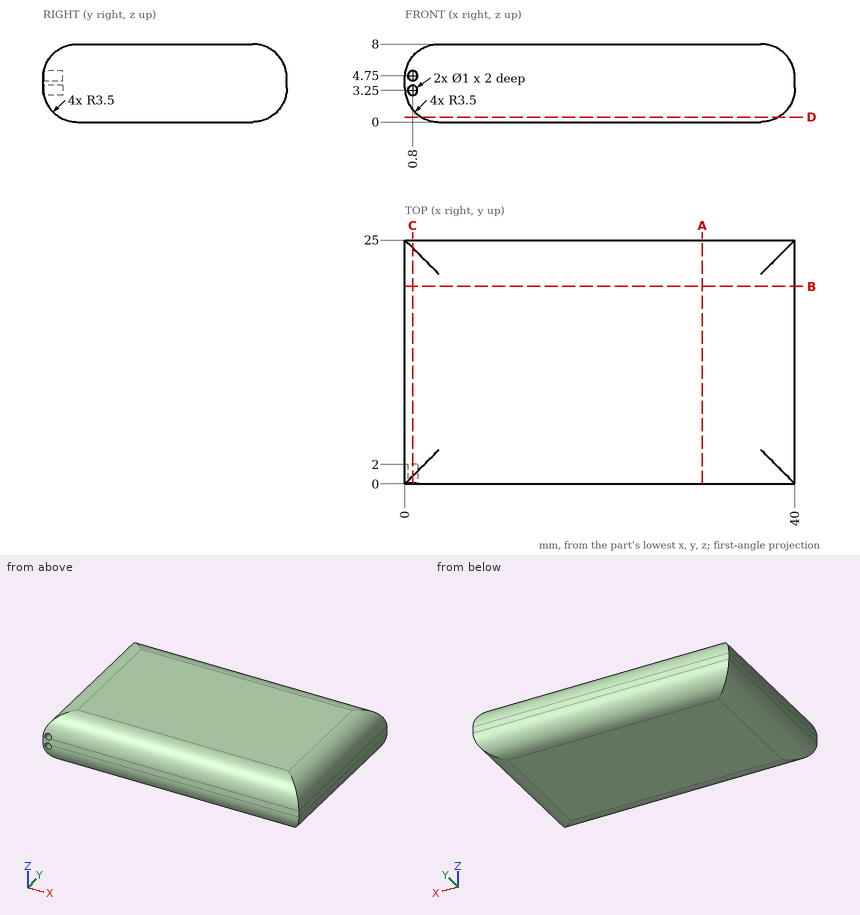
Input: dimensioned drawing with shaded views. Units: mm. Origin: part minimum x, y, z. Give positions to 0.01 mm unless a question says otherwise; leave off trailing zeros. Order: outer loops, then holes, each group sorted by start corner. A loop starts at its lowest first (then second) coordinate and runs counter-clockwise, first axis right, second up. Notation, with made-up numbers: (5.5, 16) -> (55.5, 16) arc R14 cw to (55.5, 38) -> close; hole circle Ø10 at (39, 6.25). An arc over 180 degrees is marked (long way). Answer as a JSON object with one key per item and string values.
Q1. Material intervals for probe 1 along X at (y, z) = (1.1, 3.25); probe 2 along X at (y, z) = (10.5, 3.25); probe 3 along Y at (x, z) = (8.5, 0.75), sorted ascending.
Entries:
{"probe 1": "x = 0.01 to 0.3, 1.3 to 39.99", "probe 2": "x = 0.01 to 39.99", "probe 3": "y = 1.33 to 23.67"}
Q2. First-contact query: pin 1 (2 mm diameter, centred on x = 33, z = 7, fed in from -Y). Flat tip, straight axial feed; report the tip coordinate or a pass-through.
Entries:
{"pin 1": "stops at y = 0.34"}
Q3. Section A-A (x = 30.5). Output: boundary loops of the cut face in (y, z).
Entries:
{"outline": "(0, 3.5) arc R3.5 ccw to (3.5, 0) -> (21.5, 0) arc R3.5 ccw to (25, 3.5) -> (25, 4.5) arc R3.5 ccw to (21.5, 8) -> (3.5, 8) arc R3.5 ccw to (0, 4.5) -> close"}
Q4. Section C-C (x = 0.8). Output: boundary loops of the cut face in (y, z), plus the area to 3 significant figures.
Entries:
{"outline": "(0, 3.75) -> (2, 3.75) -> (2, 2.75) -> (0.08, 2.75) arc R3.5 ccw to (0.8, 1.27) -> (24.2, 1.27) arc R3.5 ccw to (25, 3.5) -> (25, 4.5) arc R3.5 ccw to (24.2, 6.73) -> (0.8, 6.73) arc R3.5 ccw to (0.08, 5.25) -> (2, 5.25) -> (2, 4.25) -> (0, 4.25) -> close", "area": "130 mm^2"}
Q5. Section B-B (y = 20.25). Output: boundary loops of the cut face in (x, z).
Entries:
{"outline": "(0, 3.5) arc R3.5 ccw to (3.5, 0) -> (36.5, 0) arc R3.5 ccw to (40, 3.5) -> (40, 4.5) arc R3.5 ccw to (36.5, 8) -> (3.5, 8) arc R3.5 ccw to (0, 4.5) -> close"}
Q6. Section D-D (z = 0.5). Output: boundary loops of the cut face in (x, y), plus the area to 3 significant figures.
Entries:
{"outline": "(1.7, 1.7) -> (38.3, 1.7) -> (38.3, 23.3) -> (1.7, 23.3) -> close", "area": "791 mm^2"}
